Design review of the part built by this model. Coordinates are the model's own, in mm. Face numbers are marked on the shaded views. A direction names the side the tool comes from. Round coordinates to 2 decimals unless told otherwise and drop trailing zeros. Order: outer loops, then holes, each group sorted by start corner. A loop starts at its lowest first (then second) coordinate and runs counter-clockwise, first axis right, second up. Notation, with made-up numbers: (45, -3) - (84, -3) arc R31 cw to (84, 27) - close; hole circle Ø4 at (34, 30). An arc over 180 degrees is marked (long way). Write item = value, one per line.
Autodesk Inventor part; units mm, degrees
ref_plane "Work Plane1" through (0, 0, 0) normal (0, -1, 0) x (1, 0, 0)
ref_plane "Work Plane2" through (0, -250, 0) normal (0, -1, 0) x (1, 0, 0)
ref_plane "YZ Plane" through (0, 0, 0) normal (1, 0, 0) x (0, 1, 0)
sketch "Sketch1" plane through (0, 0, 0) normal (0, 1, 0) x (-1, 0, 0)
  line L0 (-650, -300) -> (650, -300)
  line L1 (650, -300) -> (650, 300)
  line L2 (650, 300) -> (-650, 300)
  line L3 (-650, 300) -> (-650, -300)
  line L4 (-650, -300) -> (650, 300) construction
  line L5 (650, -300) -> (-650, 300) construction
  line L6 (650, 300) -> (600, 300)
  line L7 (600, 250) -> (570, 250)
  line L8 (570, 220) -> (570, 90)
  line L9 (570, 90) -> (600, 90)
  line L10 (600, 90) -> (600, 250)
  line L11 (600, 250) -> (440, 250)
  line L12 (440, 250) -> (440, 220)
  line L13 (440, 220) -> (570, 220)
  line L14 (600, 220) -> (600, 250)
  line L15 (650, -300) -> (600, -300)
  line L16 (650, -250) -> (650, -300)
  line L17 (600, -250) -> (440, -250)
  line L18 (440, -250) -> (440, -220)
  line L19 (440, -220) -> (570, -220)
  line L20 (600, -220) -> (600, -250)
  line L21 (600, -250) -> (570, -250)
  line L22 (570, -220) -> (570, -90)
  line L23 (570, -90) -> (600, -90)
  line L24 (600, -90) -> (600, -250)
  line L25 (-650, 300) -> (-600, 300)
  line L26 (-650, 250) -> (-650, 300)
  line L27 (-600, 250) -> (-570, 250)
  line L28 (-570, 220) -> (-570, 90)
  line L29 (-570, 90) -> (-600, 90)
  line L30 (-600, 90) -> (-600, 250)
  line L31 (-600, 250) -> (-440, 250)
  line L32 (-440, 250) -> (-440, 220)
  line L33 (-440, 220) -> (-570, 220)
  line L34 (-600, 220) -> (-600, 250)
  line L35 (-650, -300) -> (-600, -300)
  line L36 (-650, -250) -> (-650, -300)
  line L37 (-600, -250) -> (-440, -250)
  line L38 (-440, -250) -> (-440, -220)
  line L39 (-440, -220) -> (-570, -220)
  line L40 (-600, -220) -> (-600, -250)
  line L41 (-600, -250) -> (-570, -250)
  line L42 (-570, -220) -> (-570, -90)
  line L43 (-570, -90) -> (-600, -90)
  line L44 (-600, -90) -> (-600, -250)
  point P0 (0, 0)
  dimension "d0" = 1300
  dimension "d1" = 600
  dimension "d4" = 30
  dimension "d5" = 160
  dimension "d6" = 30
  dimension "d7" = 50
  dimension "d8" = 50
  dimension "d9" = 50
  dimension "d10" = 50
  dimension "d11" = 30
  dimension "d12" = 160
  dimension "d13" = 160
  dimension "d14" = 30
extrude "Extrusion1" add sketch "Sketch1" along normal blind 60 contours L3 L2 L1 L0 | L10 L9 L8 L13 L12 L11 L7 | L17 L18 L19 L22 L23 L24 L20 | L27 L31 L32 L33 L28 L29 L30 | L40 L44 L43 L42 L39 L38 L37
ref_plane "Work Plane1" through (0, 0, 0) normal (0, -1, 0) x (1, 0, 0)
sketch "Sketch2" plane through (0, 0, 0) normal (0, -1, 0) x (1, 0, 0)
  line L0 (650, 300) -> (650, -300)
  line L1 (650, 300) -> (600, 300)
  line L2 (650, 250) -> (650, 300)
  line L3 (650, -300) -> (600, -300)
  line L4 (650, -250) -> (650, -300)
  line L5 (-650, -300) -> (-650, 300)
  line L6 (-650, -300) -> (-600, -300)
  line L7 (-650, -250) -> (-650, -300)
  line L8 (-650, 300) -> (-600, 300)
  line L9 (-650, 250) -> (-650, 300)
  line L10 (-600, -250) -> (-440, -250)
  line L11 (-440, -250) -> (-440, -220)
  line L12 (-440, -220) -> (-570, -220)
  line L13 (-600, -220) -> (-600, -250)
  line L14 (-600, -250) -> (-570, -250)
  line L15 (-570, -220) -> (-570, -90)
  line L16 (-570, -90) -> (-600, -90)
  line L17 (-600, -90) -> (-600, -250)
  line L18 (-600, 250) -> (-440, 250)
  line L19 (-440, 250) -> (-440, 220)
  line L20 (-440, 220) -> (-570, 220)
  line L21 (-600, 220) -> (-600, 250)
  line L22 (-600, 250) -> (-570, 250)
  line L23 (-570, 220) -> (-570, 90)
  line L24 (-570, 90) -> (-600, 90)
  line L25 (-600, 90) -> (-600, 250)
  line L26 (600, -250) -> (440, -250)
  line L27 (440, -250) -> (440, -220)
  line L28 (440, -220) -> (570, -220)
  line L29 (600, -220) -> (600, -250)
  line L30 (600, -250) -> (570, -250)
  line L31 (570, -220) -> (570, -90)
  line L32 (570, -90) -> (600, -90)
  line L33 (600, -90) -> (600, -250)
  line L34 (600, 250) -> (570, 250)
  line L35 (570, 220) -> (570, 90)
  line L36 (570, 90) -> (600, 90)
  line L37 (600, 90) -> (600, 250)
  line L38 (600, 250) -> (440, 250)
  line L39 (440, 250) -> (440, 220)
  line L40 (440, 220) -> (570, 220)
  line L41 (600, 220) -> (600, 250)
  point P0 (0, 0)
  dimension "d18" = 50
  dimension "d19" = 50
  dimension "d20" = 50
  dimension "d21" = 50
  dimension "d22" = 50
  dimension "d23" = 50
  dimension "d24" = 50
  dimension "d25" = 50
  dimension "d26" = 160
  dimension "d27" = 30
  dimension "d28" = 30
  dimension "d29" = 160
  dimension "d30" = 160
  dimension "d31" = 30
  dimension "d32" = 30
  dimension "d33" = 160
  dimension "d34" = 160
  dimension "d35" = 30
  dimension "d36" = 30
  dimension "d37" = 160
extrude "Extrusion2" add sketch "Sketch2" along normal blind 500
ref_plane "Work Plane2" through (0, -250, 0) normal (0, -1, 0) x (1, 0, 0)
sketch "Sketch3" plane through (0, -250, 0) normal (0, -1, 0) x (1, 0, 0)
  line L0 (570, 220) -> (-570, 220)
  line L1 (-570, 220) -> (-570, -220)
  line L2 (-570, -220) -> (570, -220)
  line L3 (570, -220) -> (570, 220)
  point P0 (0, 0)
extrude "Extrusion3" add sketch "Sketch3" along normal blind 20 and the other way blind 20
properties part number "Sto u dnevnoj sobi" material "Wood (Birch)"
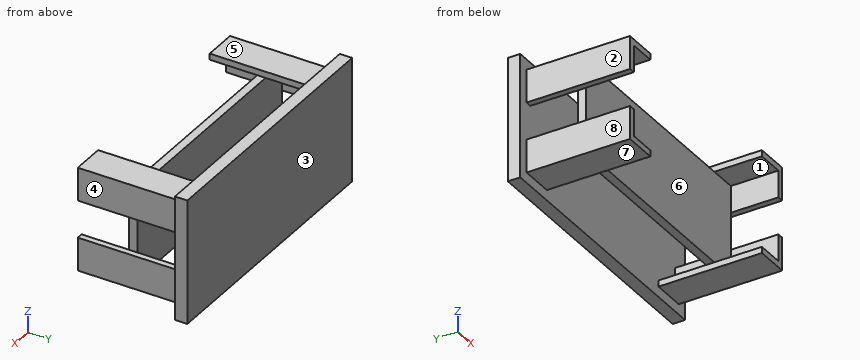
1) To check wall thickness, follow L1, parallel to X at y = -288.5, z = 160.5; L2, parallel to Y at x = -544, z = 146; L3, parallel to Z at x = -581.5, y = -214. State the ranges of each line that lie inside material, in increasing order. Write a range as from..to.
Findings:
L1 = -600..-570, 570..600
L2 = -270..-230, 0..60
L3 = -250..-90, 90..250
2) Clearance check with flat-ended pins moving along their axes: pin 1 Ø1.5 at (y, z) = (-147, -112.5) entering from +X; pin 2 Ø6 at (x, z) = (486, 87.5) entering from -Y; pin 3 Ø24 at (x, y) = (591, -277.5) entering from -Z. State where each tip first meets the part, or that it passes through.
Findings:
pin_1 = 600
pin_2 = -270
pin_3 = -250
3) For the marked faces 4, 5, 6, 7 and 8, list the 3-axis set-ups (+Z, -Z, +X, -X, +Y, -Y) from which the entire face can be reached by the end or side of a thin tool; tool diameter is ignored.
Findings:
face_4 = +Z, -Z, +X, -Y
face_5 = +Z, +X, -X, -Y
face_6 = -Y
face_7 = -Z, +X, -X, -Y
face_8 = +Z, -Z, -X, -Y
4) We need section D-D on x = 161. Write out the cut boundary in (y, z), and give its area (3 significant figures).
Findings:
outline = (-270, -220) - (-230, -220) - (-230, 220) - (-270, 220) - close; (0, -300) - (60, -300) - (60, 300) - (0, 300) - close
area = 53,600 mm^2
5) We need section B-B on y = -287. Write out the cut boundary in (x, z).
Findings:
outline = (-600, -250) - (-440, -250) - (-440, -220) - (-570, -220) - (-570, -90) - (-600, -90) - close; (-600, 90) - (-570, 90) - (-570, 220) - (-440, 220) - (-440, 250) - (-600, 250) - close; (440, -250) - (600, -250) - (600, -90) - (570, -90) - (570, -220) - (440, -220) - close; (440, 220) - (570, 220) - (570, 90) - (600, 90) - (600, 250) - (440, 250) - close
6) The part is to be moulded in two halves that separate along X. For the marked faces 1, 2 and 3, say which applies: released by +X, released by -X, zero draft, split by the parting line, or undercut.
Findings:
face_1 = undercut
face_2 = released by -X
face_3 = zero draft
7) We need section C-C on x = 503. Write out the cut boundary in (y, z), and give its area (3 significant figures).
Findings:
outline = (-500, -250) - (0, -250) - (0, -300) - (60, -300) - (60, 300) - (0, 300) - (0, 250) - (-500, 250) - (-500, 220) - (-270, 220) - (-270, -220) - (-500, -220) - close; hole (-230, -220) - (0, -220) - (0, 220) - (-230, 220) - close
area = 83,600 mm^2
8) We need section A-A on z = 26. Write out the cut boundary in (x, y), and give its area (3 significant figures).
Findings:
outline = (-650, 0) - (650, 0) - (650, 60) - (-650, 60) - close; (-570, -270) - (570, -270) - (570, -230) - (-570, -230) - close
area = 124,000 mm^2
